Design review of the part built by this model. Coordinates are the model's own, in mm. Face numbers are marked on the shaded views. A direction names the side the tool comes from. Round coordinates to 2 decimals unless told otherwise and drop trailing zeros. Loops run counter-clockwise (first coordinate to the right, second up) from the corner with the lowest first, then second, coordinate; pieces in that order, holes last. Notation, with made-up numbers: M 52,-17 L 73,-17 A22 cw 73,12 Z; hole C 5,69.5 d9. An arc over 180 degrees is marked long. Answer as CSV lines item,"result". Start each with the question number.
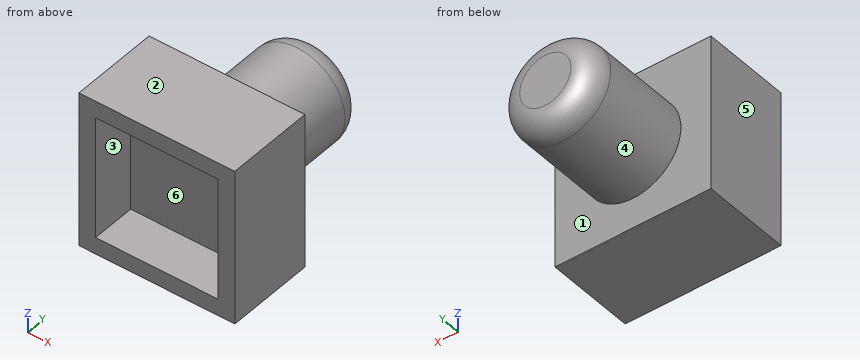
from build123d import *

# Parameters (mm, degrees)
SKETCH1_R                = 2.15
BOSS_EXTRUDE1_DEPTH      = 7
SKETCH3_W                = 7
SKETCH3_H                = 7
BOSS_EXTRUDE2_DEPTH      = 2
BOSS_EXTRUDE2_DEPTH_BACK = 2
FILLET1_R                = 1
SKETCH5_W                = 5.5
SKETCH5_H                = 5.5
CUT_EXTRUDE1_DEPTH       = 2


with BuildPart() as part:
    # Sketch1 → Boss-Extrude1 (new body)
    with BuildSketch(Plane(origin=(0, 0, 0), x_dir=(1, 0, 0), z_dir=(0, 1, 0))):
        Circle(SKETCH1_R)
    extrude(amount=BOSS_EXTRUDE1_DEPTH)

    # Sketch3 → Boss-Extrude2 (add, two sides)
    with BuildSketch(Plane.XZ) as boss_extrude2_sk:
        Rectangle(SKETCH3_W, SKETCH3_H)
    extrude(amount=BOSS_EXTRUDE2_DEPTH)
    extrude(boss_extrude2_sk.sketch, amount=-BOSS_EXTRUDE2_DEPTH_BACK)

    # Fillet1
    fillet1_edges = [part.edges().sort_by_distance(p)[0] for p in [
        (-2.15, 7, 0),
    ]]
    fillet(fillet1_edges, radius=FILLET1_R)

    # Sketch5 → Cut-Extrude1 (cut)
    with BuildSketch(Plane.XZ.offset(2)):
        Rectangle(SKETCH5_W, SKETCH5_H)
    extrude(amount=-CUT_EXTRUDE1_DEPTH, mode=Mode.SUBTRACT)


solid = part.part
Item 1: Consider section C-C, the plane z = 0. Write out the cut boundary in (x, y), then the cut area to 3 significant figures.
Item 2: To check wall thickness, follow line 1 (Z direction, x = -2.5, y = -1.5); line 2 (Y direction, x = 2.5, z = -2.5). State the ranges of each line that lie inside material, in increasing order.
Item 3: Insertion check: pin 1 Ø1.5 at (x, y) = (-0.5, 3) entering from -Z. The pin has a flat end and moves straight along its axis. Give the tip position at first contact, or say it passes through.
Item 4: Consider section A-A, the plane y = -0.75. Write out the cut boundary in (x, z).
Item 5: Consider section B-B, the plane x = 0. Write out the cut boundary in (y, z), then the cut area to 3 significant figures.
Item 6: Tool access review of the marked faces 1, 2 and 3: name each direction out of +Z, -Z, +X, -X, +Y, -Y from which nothing blocks a thin tool from reaching the whole face with its end or side.
Item 7: The part is to be moulded in two halves that separate along X. For the marked faces 4, 5 and 6, say which applies: +X half, -X half, draft (parallel to the pull), parting line (faces both ways), or undercut.
Item 8: Consider section D-D, the plane y = 5.75. Write out the cut boundary in (x, z), then the cut area to 3 significant figures.
Found:
1,outline,"M -3.5,-2 L -2.75,-2 L -2.75,0 L 2.75,0 L 2.75,-2 L 3.5,-2 L 3.5,2 L 2.15,2 L 2.15,6 A1 ccw 1.15,7 L -1.15,7 A1 ccw -2.15,6 L -2.15,2 L -3.5,2 Z"
1,area,"38.1 mm^2"
2,line 1,"z = -3.5 to -2.75, 2.75 to 3.5"
2,line 2,"y = 0 to 2"
3,pin 1,"stops at z = -2.15"
4,outline,"M -3.5,-3.5 L 3.5,-3.5 L 3.5,3.5 L -3.5,3.5 Z; hole M -2.75,-2.75 L 2.75,-2.75 L 2.75,2.75 L -2.75,2.75 Z"
5,outline,"M -2,-3.5 L 2,-3.5 L 2,-2.15 L 6,-2.15 A1 ccw 7,-1.15 L 7,1.15 A1 ccw 6,2.15 L 2,2.15 L 2,3.5 L -2,3.5 L -2,2.75 L 0,2.75 L 0,-2.75 L -2,-2.75 Z"
5,area,"38.1 mm^2"
6,face 1,"+Y"
6,face 2,"+Z, +X, -X, +Y, -Y"
6,face 3,"-Y"
7,face 4,"parting line"
7,face 5,"-X half"
7,face 6,"undercut"
8,outline,"C 0,0 d4.3"
8,area,"14.5 mm^2"
